Verification items for this drawing (mm, ordinates from the low corner). A direction names the side the tool comes from. Coordinates: 2 decimals unless noted, no trailing zeros. Loops run counter-clockwise (first coordinate to the right, second up) from the corner with the lowest first, then second, coordinate; pieces in that order, holes last. Notation, with made-up numbers: (36.25, 49.5) -> (56.25, 49.5) arc R25 ccw to (56.25, 70.5) -> close; hole circle Ø11 at (19.25, 79). An arc over 180 degrees is marked (long way). Write item = value, one per line.
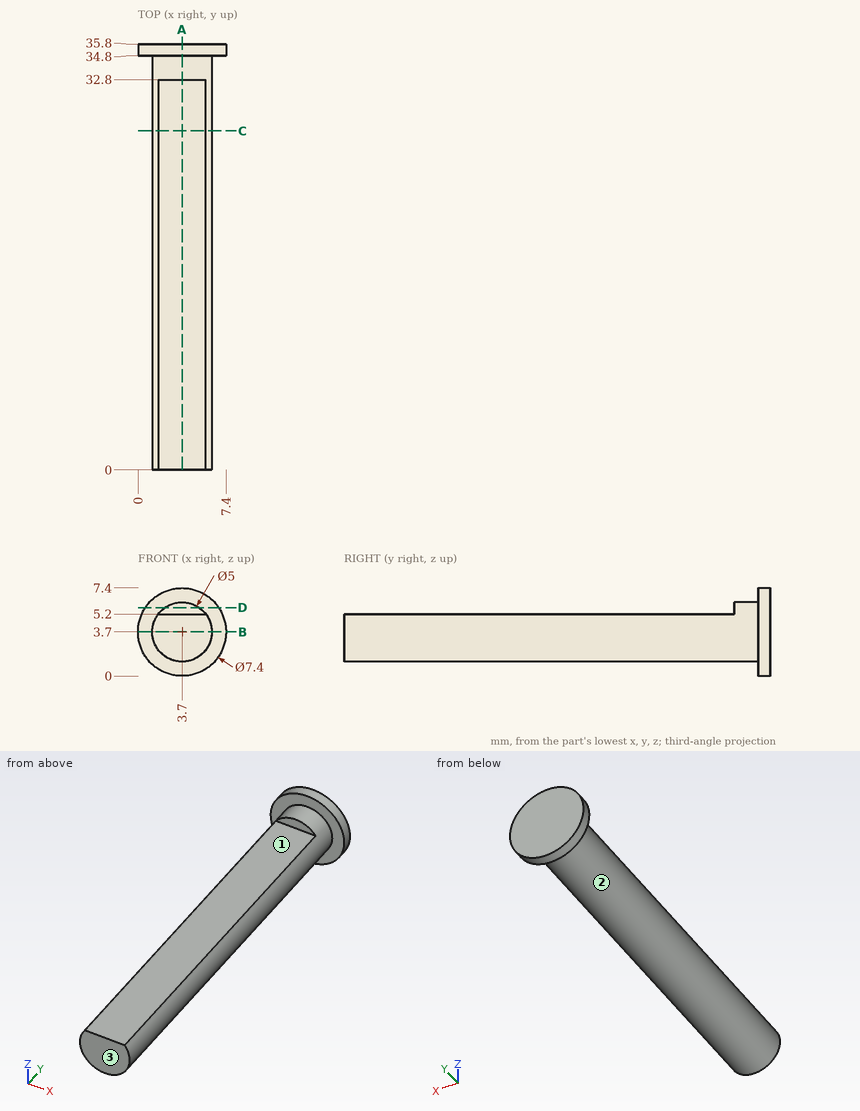
1) Material ranges on line 1 (Y direction, x = 3.5, z = 6.25); line 2 (Y direction, x = 3, z = 5.25); line 3 (Z direction, x = 3.5, y = 12), recorded low to high.
Ans:
line_1 = 34.8 to 35.8
line_2 = 32.8 to 35.8
line_3 = 1.21 to 5.2
2) Sectioned sample at C-C, the plane y = 28.5. Record the cut outline in (x, z).
Ans:
outline = (1.7, 5.2) arc R2.5 ccw (long way) to (5.7, 5.2) -> close
3) Tool access check on the marked faces 1, 2 and 3. Record the directions out of +Z, -Z, +X, -X, +Y, -Y that give a thin tool (end or side, any length) a straight path to the whole face; none if there is none.
Ans:
face_1 = +Z, +X, -X, -Y
face_2 = -Y
face_3 = +Z, -Z, +X, -X, -Y
4) Sectioned sample at A-A, the plane x = 3.7. Record the cut outline in (y, z).
Ans:
outline = (0, 1.2) -> (34.8, 1.2) -> (34.8, 0) -> (35.8, 0) -> (35.8, 7.4) -> (34.8, 7.4) -> (34.8, 6.2) -> (32.8, 6.2) -> (32.8, 5.2) -> (0, 5.2) -> close
5) Sectioned sample at D-D, the plane z = 5.75. Record the cut outline in (x, y).
Ans:
outline = (0.62, 34.8) -> (2.27, 34.8) -> (2.27, 32.8) -> (5.13, 32.8) -> (5.13, 34.8) -> (6.78, 34.8) -> (6.78, 35.8) -> (0.62, 35.8) -> close
6) Sectioned sample at B-B, the plane z = 3.7. Record the cut outline in (x, y), plus the area to 3 significant figures.
Ans:
outline = (0, 34.8) -> (1.2, 34.8) -> (1.2, 0) -> (6.2, 0) -> (6.2, 34.8) -> (7.4, 34.8) -> (7.4, 35.8) -> (0, 35.8) -> close
area = 181 mm2
7) Depth check by flat-ended pin: pin 1 Ø3 at (x, y) = (4, 20.5) entering from +Z; pin 2 Ø2 at (x, y) = (2.5, 30) entering from -Z; pin 3 Ø4 at (y, z) = (8.5, 3) entering from -X. Enter the tip coordinate at first touch or a pass-through.
Ans:
pin_1 = 5.2
pin_2 = 1.21
pin_3 = 1.2
